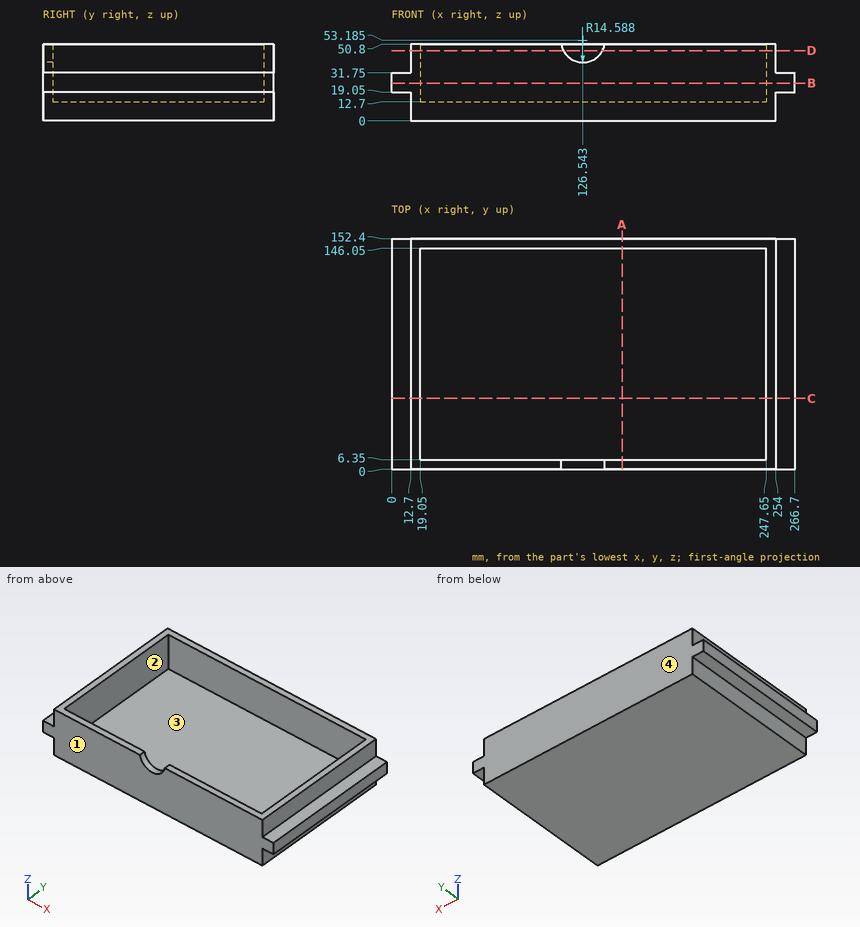
Input: dimensioned drawing with shaded views. Units: mm. Origin: part minimum x, y, z. A direction names the side the tool comes from. Coordinates: 2 decimals unless noted, no trailing zeros. Order: outer loops, then holes, each group sorted by start corner. A loop starts at its lowest first (then second) coordinate and runs counter-clockwise, first axis right, second up.
Item 1: Section query A-A (x = 152.5). Output: boundary loops of the cut face in (y, z), then the cut area to 3 significant figures.
Answer:
outline: (0, 0) - (152.4, 0) - (152.4, 50.8) - (146.05, 50.8) - (146.05, 12.7) - (6.35, 12.7) - (6.35, 50.8) - (0, 50.8) - close
area: 2,420 mm2
Item 2: Draft query along X for the marked faces 1 and 2. Return one class per face: released by +X, released by -X, zero draft, split by the parting line, or undercut.
Answer:
face 1: zero draft
face 2: undercut
Item 3: Access query for the marked faces 3 and 4. Directions: +Z, -Z, +X, -X, +Y, -Y. A direction counts if a zero-diameter tool reaches every point of the face in a straight line with its end or side. Return the directions, or none.
Answer:
face 3: +Z
face 4: +Z, -Z, +X, -X, +Y
Item 4: Section query B-B (z = 25). Output: boundary loops of the cut face in (x, y).
Answer:
outline: (0, 0) - (266.7, 0) - (266.7, 152.4) - (0, 152.4) - close; hole (19.05, 6.35) - (247.65, 6.35) - (247.65, 146.05) - (19.05, 146.05) - close
Item 5: Material intervals for line 1 along Y through (x, z) = (208.5, 25); line 2 along X through (y, z) = (143, 35), sorted ascending.
Answer:
line 1: y = 0 to 6.35, 146.05 to 152.4
line 2: x = 12.7 to 19.05, 247.65 to 254
Item 6: Contact query for flat-ended pins moving along their axis: P1, Ø10, axis at x = 4, y = 45, coming from the +Z side; P2, Ø9.5, axis at y = 98, z = 45.5, coming from the +X side; P3, Ø9.5, axis at y = 68, z = 8.5, coming from the -X side. Output: stop coordinate, or through.
Answer:
P1: stops at z = 31.75
P2: stops at x = 254
P3: stops at x = 12.7
Item 7: Section query C-C (y = 47). Output: boundary loops of the cut face in (x, z), then the cut area to 3 significant figures.
Answer:
outline: (0, 19.05) - (12.7, 19.05) - (12.7, 0) - (254, 0) - (254, 19.05) - (266.7, 19.05) - (266.7, 31.75) - (254, 31.75) - (254, 50.8) - (247.65, 50.8) - (247.65, 12.7) - (19.05, 12.7) - (19.05, 50.8) - (12.7, 50.8) - (12.7, 31.75) - (0, 31.75) - close
area: 3,870 mm2
Item 8: Section query D-D (z = 46.5). Output: boundary loops of the cut face in (x, y).
Answer:
outline: (12.7, 0) - (113.58, 0) - (113.58, 6.35) - (19.05, 6.35) - (19.05, 146.05) - (247.65, 146.05) - (247.65, 6.35) - (139.51, 6.35) - (139.51, 0) - (254, 0) - (254, 152.4) - (12.7, 152.4) - close
